Build history of the part. All positions in model axes, mm. Round coordinates to 2 decimals unless told otherwise and drop trailing zeros. Loops run counter-clockwise (first coordinate to the right, second up) from the corner with the lowest first, then second, coordinate; pieces in that order, holes last.
from build123d import *

# Parameters (mm, degrees)
SKETCH2_R            = 3.175
BOSS_EXTRUDE1_DEPTH  = 10
FILLET1_R            = 10
FILLET1_OF_MIRROR1_R = 10


with BuildPart() as part:
    # Sketch2 → Boss-Extrude1 (new body)
    with BuildSketch(Plane.XY):
        with BuildLine():
            Line((320.613470585, -114.844314923), (222.622994392, -300))
            Line((222.622994392, -300), (201, -300))
            ThreePointArc((201, -300), (199.292893219, -299.292893219), (200, -301))
            Line((200, -301), (200, -338.582))
            Line((200, -338.582), (0, -338.582))
            Line((0, -338.582), (0, -236.982))
            Line((0, -236.982), (87.523, -236.982))
            Line((87.523, -236.982), (87.523, -286.782))
            ThreePointArc((87.523, -286.782), (86.815893219, -288.489106781), (88.523, -287.782))
            Line((88.523, -287.782), (99.477, -287.782))
            ThreePointArc((99.477, -287.782), (101.184106781, -288.489106781), (100.477, -286.782))
            Line((100.477, -286.782), (100.477, -236.982))
            Line((100.477, -236.982), (212.208138071, -236.982))
            ThreePointArc((212.208138071, -236.982), (214.858618264, -235.977822883), (216.178322678, -233.469477374))
            Line((216.178322678, -233.469477374), (222.957537911, -178.2572))
            Line((222.957537911, -178.2572), (242.173347705, -178.2572))
            ThreePointArc((242.173347705, -178.2572), (244.744498144, -177.321377772), (246.112578717, -174.951792711))
            Line((246.112578717, -174.951792711), (255.875555496, -119.5832))
            Line((255.875555496, -119.5832), (269.308394175, -119.5832))
            ThreePointArc((269.308394175, -119.5832), (271.958874368, -118.579022883), (273.278578782, -116.070677374))
            Line((273.278578782, -116.070677374), (279.630331697, -64.339801211))
            Line((279.630331697, -64.339801211), (320.613470585, -64.044314923))
            Line((320.613470585, -64.044314923), (320.613470585, -114.844314923))
        make_face()
        with Locations((275, -150)):
            Circle(SKETCH2_R, mode=Mode.SUBTRACT)
        with Locations((242.256504613, -211.869730158)):
            Circle(SKETCH2_R, mode=Mode.SUBTRACT)
    boss_extrude1 = extrude(amount=BOSS_EXTRUDE1_DEPTH)

    # Fillet1
    fillet1_edges = [part.edges().sort_by_distance(p)[0] for p in [
        (222.957537911, -178.2572, 5),
        (255.875555496, -119.5832, 5),
    ]]
    fillet(fillet1_edges, radius=FILLET1_R)

    # Mirror1: Boss-Extrude1 across plane
    add(boss_extrude1.mirror(Plane(origin=(0, 0, 10), x_dir=(0, 0, 1), z_dir=(1, 0, 0))))

    # Fillet1 of Mirror1
    fillet1_of_mirror1_edges = [part.edges().sort_by_distance(p)[0] for p in [
        (-222.957537911, -178.2572, 5),
        (-255.875555496, -119.5832, 5),
    ]]
    fillet(fillet1_of_mirror1_edges, radius=FILLET1_OF_MIRROR1_R)


solid = part.part
(1) Slice it at A-A on y = -202.5. List the corners of the cut face in (x, z), plus the area to 3 significant figures.
Responses:
outline: (-274.22, 0) - (-219.98, 0) - (-219.98, 10) - (-274.22, 10) - close; (219.98, 0) - (274.22, 0) - (274.22, 10) - (219.98, 10) - close
area: 1,080 mm2
(2) Slice it at D-D on z = 3.5. Count the separate pieces of the cut face and the enclosed holes in it, plus the area to 3 significant figures.
Responses:
separate pieces: 1
enclosed holes: 4
area: 61,200 mm2
(3) Slice it at C-C on x = 18.5. List the corners of the cut face in (y, z).
Responses:
outline: (-338.58, 0) - (-236.98, 0) - (-236.98, 10) - (-338.58, 10) - close
(4) Slice it at B-B on y = -320. List the corners of the cut face in (x, z), plus the area to 3 significant figures.
Responses:
outline: (-200, 0) - (200, 0) - (200, 10) - (-200, 10) - close
area: 4,000 mm2
(5) Probe line 1 (X direction, y = -238, z = 8); line 2 (X direction, y = -244.5, z = 2); line 3 (Y direction, x = -198.5, z = 0.5). List the from-to ranges inside material, lowest first.
Responses:
line 1: x = -255.44 to -100.48, -87.52 to 87.52, 100.48 to 255.44
line 2: x = -252 to -100.48, -87.52 to 87.52, 100.48 to 252
line 3: y = -338.58 to -236.98
(6) Pin check, flat tips, straight feed: P1, Ø5.5, axis at x = 266.5, z = 6.5, coming from the +Y side; P2, Ø5, axis at x = -237.5, z = 6, coming from the +Y side; P3, Ø1, axis at y = -211.5, z = 8.5, coming from the -X side. Stop position of each tip, or through.
Responses:
P1: stops at y = -119.58
P2: stops at y = -178.26
P3: stops at x = -269.72
